Check sheet for the modelled part. Datum: model origin and axes. Units: mm. Face numbers are marked on the shaded views. A direction names the side the tool comes from. Coordinates: 2 decimals unless noted, no trailing zeros. Loops run counter-clockwise (first coordinate to the right, second up) from the corner with the lowest first, then second, coordinate; pieces in that order, holes last. Notation, with made-up numbers: (21.25, 83.5) -> (72.25, 83.5) arc R7 ccw to (72.25, 94.5) -> close; hole circle Ø11 at (63, 20). An arc over 180 degrees is marked (long way). Use CSV: the item, a comma, the result in double quotes. Start each with the question number.
1. Release check for a two-part mould opening along Y. For the marked faces 1, 2 and 3 record: pulls with the +Y half, pulls with the -Y half, needs draft (parallel to the pull), parting line crosses it, or undercut.
2. Sectioned sample at D-D, the plane y = 12.5. Record the cut outline in (x, z).
3. Thickness scan on L1, parallel to X at y = 38.1, z = 5.25; L2, parallel to Y at x = -6, z = 41; L3, parallel to Y at x = -25, z = 7. Record the ranges inside material, lowest first.
4. Sectioned sample at B-B, the plane z = 52. Record the cut outline in (x, y).
5. Gauge pin test, flat end, axial feed: pin 1 (6 mm diameter, centred on x = -40, y = -34, fed in from +Z). Record the tip position at first contact, or that the pin passes through.
6. Sectioned sample at A-A, the plane x = -25.4. Record the cut outline in (y, z), and give its area (3 significant figures).
7. Set-up check for the marked faces 4 and 5: record each of +Z, -Z, +X, -X, +Y, -Y from which the full face is reachable in a straight line by a thin tool's end or side.
8. Sectioned sample at C-C, the plane y = 38.1. Record the cut outline in (x, z).
```python
from build123d import *

# Parameters (mm, degrees)
F0_W     = 127
F0_H     = 127
F1_DEPTH = 76.2
F2_W     = 116.84
F2_H     = 116.84
F3_DEPTH = 66.04
F4_R     = 6.35
F5_DEPTH = 76.201


with BuildPart() as f1:
    # F0 (on Top) → F1 (new body)
    with BuildSketch(Plane.XY):
        Rectangle(F0_W, F0_H)
    extrude(amount=F1_DEPTH)

    # F2 (on face) → F3 (cut)
    with BuildSketch(Plane.XY.offset(76.2)):
        Rectangle(F2_W, F2_H)
    extrude(amount=-F3_DEPTH, mode=Mode.SUBTRACT)

    # F4 (on face) → F5 (cut, through all)
    with BuildSketch(Plane(origin=(0, 0, 0), x_dir=(1, 0, 0), z_dir=(0, 0, -1))):
        with Locations((-25.4, -38.1)):
            Circle(F4_R)
    extrude(amount=-F5_DEPTH, mode=Mode.SUBTRACT)


solid = f1.part
```
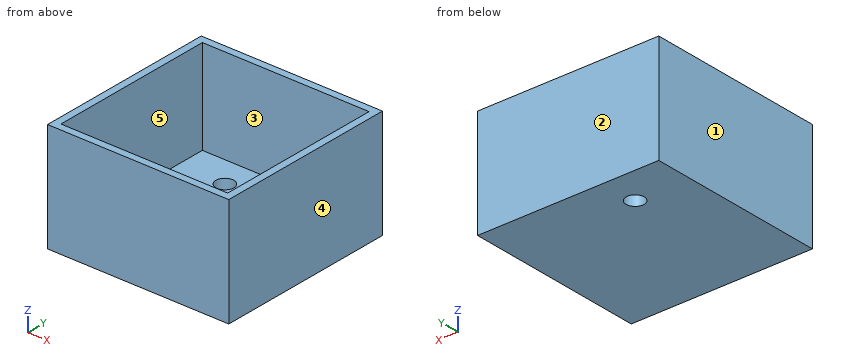
Completed:
1,face 1,"needs draft"
1,face 2,"pulls with the +Y half"
1,face 3,"undercut"
2,outline,"(-63.5, 0) -> (63.5, 0) -> (63.5, 76.2) -> (58.42, 76.2) -> (58.42, 10.16) -> (-58.42, 10.16) -> (-58.42, 76.2) -> (-63.5, 76.2) -> close"
3,L1,"-63.5 to -31.75, -19.05 to 63.5"
3,L2,"-63.5 to -58.42, 58.42 to 63.5"
3,L3,"-63.5 to 31.76, 44.44 to 63.5"
4,outline,"(-63.5, -63.5) -> (63.5, -63.5) -> (63.5, 63.5) -> (-63.5, 63.5) -> close; hole (-58.42, -58.42) -> (58.42, -58.42) -> (58.42, 58.42) -> (-58.42, 58.42) -> close"
5,pin 1,"z = 10.16"
6,outline,"(-63.5, 0) -> (31.75, 0) -> (31.75, 10.16) -> (-58.42, 10.16) -> (-58.42, 76.2) -> (-63.5, 76.2) -> close; (44.45, 0) -> (63.5, 0) -> (63.5, 76.2) -> (58.42, 76.2) -> (58.42, 10.16) -> (44.45, 10.16) -> close"
6,area,"1,830 mm²"
7,face 4,"+Z, -Z, +X, +Y, -Y"
7,face 5,"+Z"
8,outline,"(-63.5, 0) -> (-31.75, 0) -> (-31.75, 10.16) -> (-58.42, 10.16) -> (-58.42, 76.2) -> (-63.5, 76.2) -> close; (-19.05, 0) -> (63.5, 0) -> (63.5, 76.2) -> (58.42, 76.2) -> (58.42, 10.16) -> (-19.05, 10.16) -> close"
